The figure shows three views and two pictorial views of one solid part (mm, origin at its lowest corner). Answer the questions. A direction names the side the tool comes from. Coordinates: 2 decimals unless noted, no trailing zeros. Order: outer loops, then holes, each group sorted by start corner. A loop starts at its lowest first (then second) coordinate and runs counter-clockwise, first axis right, second up.
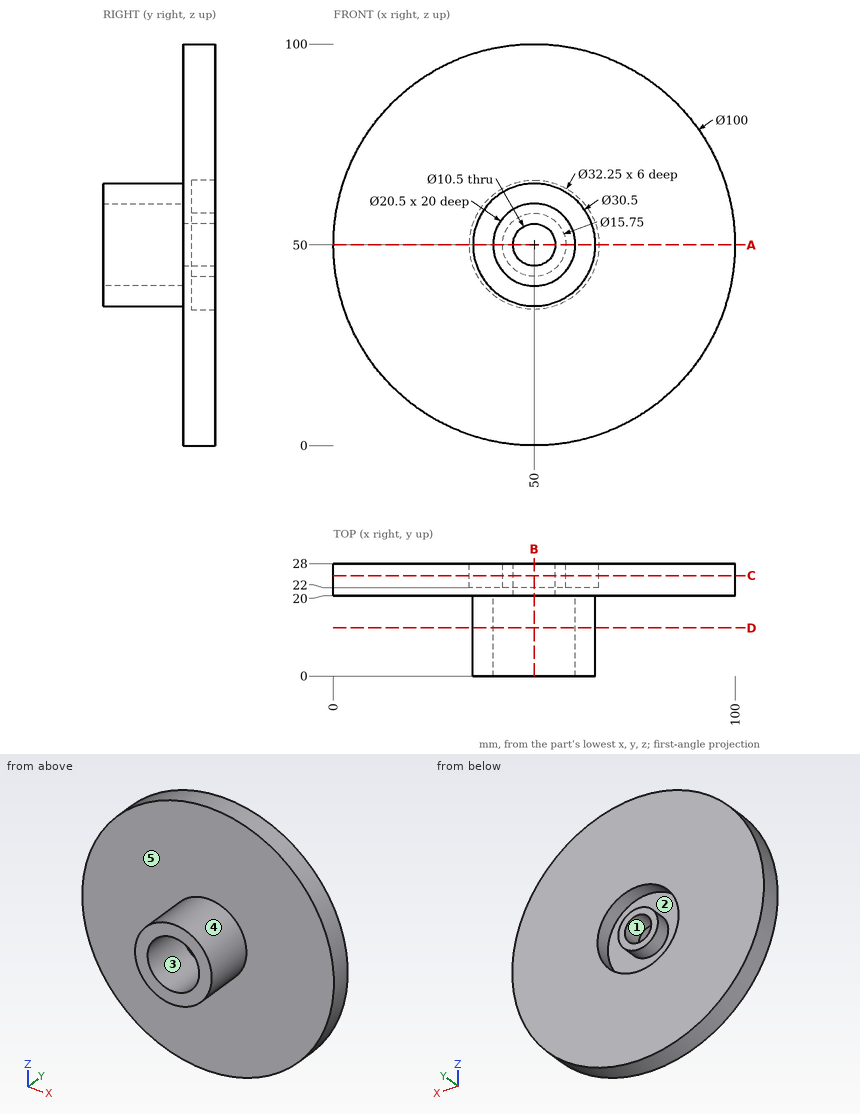
1) A cutting plane is placed at C-C, the plane y = 25. Write down the section's boundary in (x, z) (3 decimals), plus the area to 3 significant figures.
2) A cutting plane is placed at B-B, the plane x = 50. Write down the section's boundary in (y, z) (3 decimals).
3) For the marked faces 1 and 2, determine the directions among +Z, -Z, +X, -X, +Y, -Y from which every point of the face is accessible in a straight line to the end or side of a thin tool.
4) The mould has two halves that part along X. Classify the marked faces 3, 4 and 5: released by +X, released by -X, zero draft, split by the parting line, or undercut.
5) Each of these flat-tipped pins is pushed along its axis until it touches: P1, Ø10, axis at y = 9.5, z = 47, coming from the -X side; P2, Ø6, axis at x = 53, z = 52, coming from the -Y side; P3, Ø23.5, axis at x = 50, z = 50, coming from the +Y side; P4, Ø6, axis at x = 87, y = 21, coming from the -Z side. Where does it stop, or does it pass through?
6) Straight lines are drawn through the part: probe 1 along X at (y, z) = (25.75, 50) (3 decimals); probe 2 along Y at (x, z) = (65, 37.5); probe 3 along Z at (x, y) = (47, 18.5). For each, find the intervals that lie inside material, in ascending order.
7) A cutting plane is placed at D-D, the plane y = 12. Write down the section's boundary in (x, z).
8) A cutting plane is placed at A-A, the plane z = 50. Write down the section's boundary in (x, y) (3 decimals).
Working result:
1. outline: circle Ø100 at (50, 50); circle Ø15.75 at (50, 50); hole circle Ø32.25 at (50, 50); hole circle Ø10.5 at (50, 50)
1. area: 7,150 mm2
2. outline: (0, 34.75) - (20, 34.75) - (20, 0) - (28, 0) - (28, 33.875) - (22, 33.875) - (22, 42.125) - (28, 42.125) - (28, 44.75) - (20, 44.75) - (20, 39.75) - (0, 39.75) - close; (0, 60.25) - (20, 60.25) - (20, 55.25) - (28, 55.25) - (28, 57.875) - (22, 57.875) - (22, 66.125) - (28, 66.125) - (28, 100) - (20, 100) - (20, 65.25) - (0, 65.25) - close
3. face 1: +Y, -Y
3. face 2: +Y
4. face 3: undercut
4. face 4: split by the parting line
4. face 5: zero draft
5. P1: stops at x = 34.75
5. P2: stops at y = 20
5. P3: stops at y = 28
5. P4: stops at z = 13.34
6. probe 1: x = 0 to 33.875, 42.125 to 44.75, 55.25 to 57.875, 66.125 to 100
6. probe 2: y = 20 to 28
6. probe 3: z = 35.05 to 40.2, 59.8 to 64.95
7. outline: circle Ø30.5 at (50, 50); hole circle Ø20.5 at (50, 50)
8. outline: (0, 20) - (34.75, 20) - (34.75, 0) - (39.75, 0) - (39.75, 20) - (44.75, 20) - (44.75, 28) - (42.125, 28) - (42.125, 22) - (33.875, 22) - (33.875, 28) - (0, 28) - close; (55.25, 20) - (60.25, 20) - (60.25, 0) - (65.25, 0) - (65.25, 20) - (100, 20) - (100, 28) - (66.125, 28) - (66.125, 22) - (57.875, 22) - (57.875, 28) - (55.25, 28) - close
